Model file for the job. Use its own axes, mm. Face numbers are marked on the shaded views. A direction names the side the tool comes from. Round coordinates to 2 decimals unless told otherwise and drop trailing zeros. Write each loop counter-clockwise with the first axis right and the second up, starting at its lowest first coordinate (ties: lowest second). Pieces come first, ordered by that corner, then holes.
```python
from build123d import *
from OCP.BRepFilletAPI import BRepFilletAPI_MakeFillet

# Parameters (mm, degrees)
SKETCH7_R           = 5
BOSS_EXTRUDE2_DEPTH = 2.5
FILLET2_R1          = 5
FILLET2_R2          = 15


with BuildPart() as part:
    # Sketch4 → Revolve1 (revolve)
    with BuildSketch(Plane.XY, mode=Mode.PRIVATE) as revolve1_sk:
        Polygon((5, 5), (5, -5), (6, -5), (6, -25), (15, -25), (15, 25), (6, 25), (6, 5), align=None)
    revolve(revolve1_sk.sketch.rotate(Axis((0, 25, 0), (0, -1, 0)), 90), axis=Axis((0, 25, 0), (0, -1, 0)))

    # Sketch7 → Boss-Extrude2 (add, symmetric)
    with BuildSketch(Plane(origin=(0, 0, 0), x_dir=(1, 0, 0), z_dir=(0, 1, 0))):
        with BuildLine():
            Line((-15, -12.5), (-15, -129.126781955))
            Line((-15, -129.126781955), (37.082039325, -129.126781955))
            ThreePointArc((37.082039325, -129.126781955), (52.082039325, -114.126781955), (37.082039325, -99.126781955))
            Line((37.082039325, -99.126781955), (15, -99.126781955))
            Line((15, -99.126781955), (15, 0))
            ThreePointArc((15, 0), (7.093185827, -13.216910184), (-8.291561976, -12.5))
            Line((-8.291561976, -12.5), (-15, -12.5))
        make_face()
        with Locations(Location((37.082039325, -114.126781955, 0), (0, 0, 270))):
            Circle(SKETCH7_R, mode=Mode.SUBTRACT)
    extrude(amount=BOSS_EXTRUDE2_DEPTH, both=True)

    # Fillet2: one fillet with a radius per group of edges: ONE call of the kernel's fillet builder (fillet() takes one radius for all edges)
    fillet2_edges_1 = [part.edges().sort_by_distance(p)[0] for p in [
        (15, 0, 99.126781955),
    ]]
    fillet2_edges_2 = [part.edges().sort_by_distance(p)[0] for p in [
        (-15, 0, 129.126781955),
    ]]
    fillet2 = BRepFilletAPI_MakeFillet(part.part.solid().wrapped)
    for e in fillet2_edges_1:
        fillet2.Add(FILLET2_R1, e.wrapped)
    for e in fillet2_edges_2:
        fillet2.Add(FILLET2_R2, e.wrapped)
    add(Compound.cast(fillet2.Shape()), mode=Mode.REPLACE)


solid = part.part
```
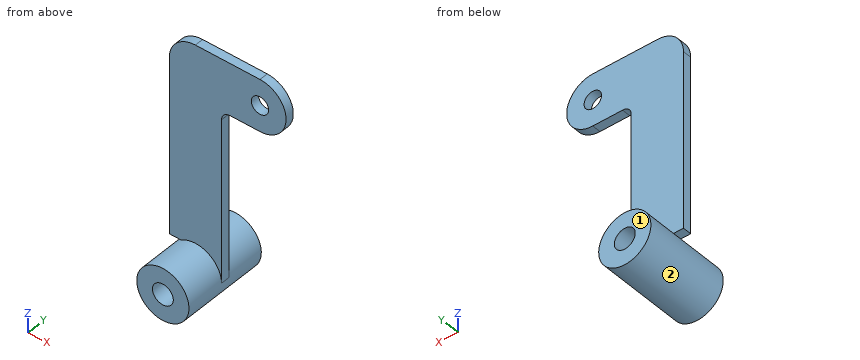
1) Cut at C-C on z = 47.5. List the corners of the cut face in (x, y), and give its area (3 significant figures).
2) Which spindle directions (+Z, -Z, +X, -X, +Y, -Y) get a long thin tool onto all of the face, cutting with end or side? Do the marked faces 1 and 2. Say none if no direction does.
3) Cut at B-B on x = 28. List the corners of the cut face in (y, z), and give its area (3 significant figures).
4) Flat gauge pins, fed straight in: pin 1 Ø5.5 at (x, y) = (28.5, 1) entering from -Z; pin 2 Ø9.5 at (x, z) = (-0.5, -1.5) entering from +Y; pin 3 Ø4 at (x, z) = (16.5, 108) entering from +Y; pin 4 Ø2.5 at (y, z) = (-1, 68) entering from +X. Where does each tip first touch, or does it go through?
5) Wall check: probe 1 along X at (y, z) = (6, 0); probe 2 along X at (y, z) = (-2, 0); probe 3 along Y at (x, z) = (0, 68). Give the ranges that are in metal, low to high.
6) Cut at A-A on y = 18.5. List the corners of the cut face in (x, z).
Result sheet:
1. outline: (-15, -2.5) - (15, -2.5) - (15, 2.5) - (-15, 2.5) - close
1. area: 150 mm2
2. face 1: +Z, -Z, +X, -X, +Y
2. face 2: none
3. outline: (-2.5, 99.13) - (2.5, 99.13) - (2.5, 129.13) - (-2.5, 129.13) - close
3. area: 150 mm2
4. pin 1: stops at z = 99.13
4. pin 2: stops at y = 25
4. pin 3: stops at y = 2.5
4. pin 4: stops at x = 15
5. probe 1: x = -15 to -6, 6 to 15
5. probe 2: x = -15 to -5, 5 to 15
5. probe 3: y = -2.5 to 2.5
6. outline: circle Ø30 at (0, 0); hole circle Ø12 at (0, 0)
